Can you work these out from the drawing? Everything is in mm from the part's minimum corner. A direction names the side the tool comes from. Round coordinates to 2 decimals unless told otherwise and drop trailing zeros. Write each loop counter-clockwise with the first axis right and the second up, starting at its lowest first coordinate (ties: lowest second). Pieces come first, ordered by that corner, then holes. Notation, with made-up numbers: (-3, 47) -> (2, 47) arc R12 ccw to (2, 53) -> close; hole circle Ø11 at (30.25, 12.5). An arc over 180 degrees is marked (long way). Answer as CSV lines item,"result". Start each with the question number.
Q1. For the marked faces 1 and 2, which set-ups out of +Z, -Z, +X, -X, +Y, -Y let a thin tool reach every point of the face, with its end or its side?
Q2. Imagine slicing it at B-B on x = 10.5. Please give me the cut outline in (y, z).
Q3. Imagine slicing it at C-C on z = 5.25. Please give me the cut outline in (x, y).
Q4. Imagine slicing it at A-A on y = 2.25. Please give me the cut outline in (x, z).
Q5. If I drill on line 1 (Z direction, x = 5.5, y = 10); line 2 (X direction, y = 17.5, z = 2.5); line 3 (Z direction, x = 2.25, y = 3.75) (1 decimal), over which ranges is the centre line in solid material (lowest first)? Write a range as [from, to].
Q6. Will these pins go through, and if not, where does the flat tip stop? pin 1 Ø4.5 at (y, z) = (7, 6) entering from +X; pin 2 Ø1.5 at (x, y) = (8.5, 2.5) entering from -Z.
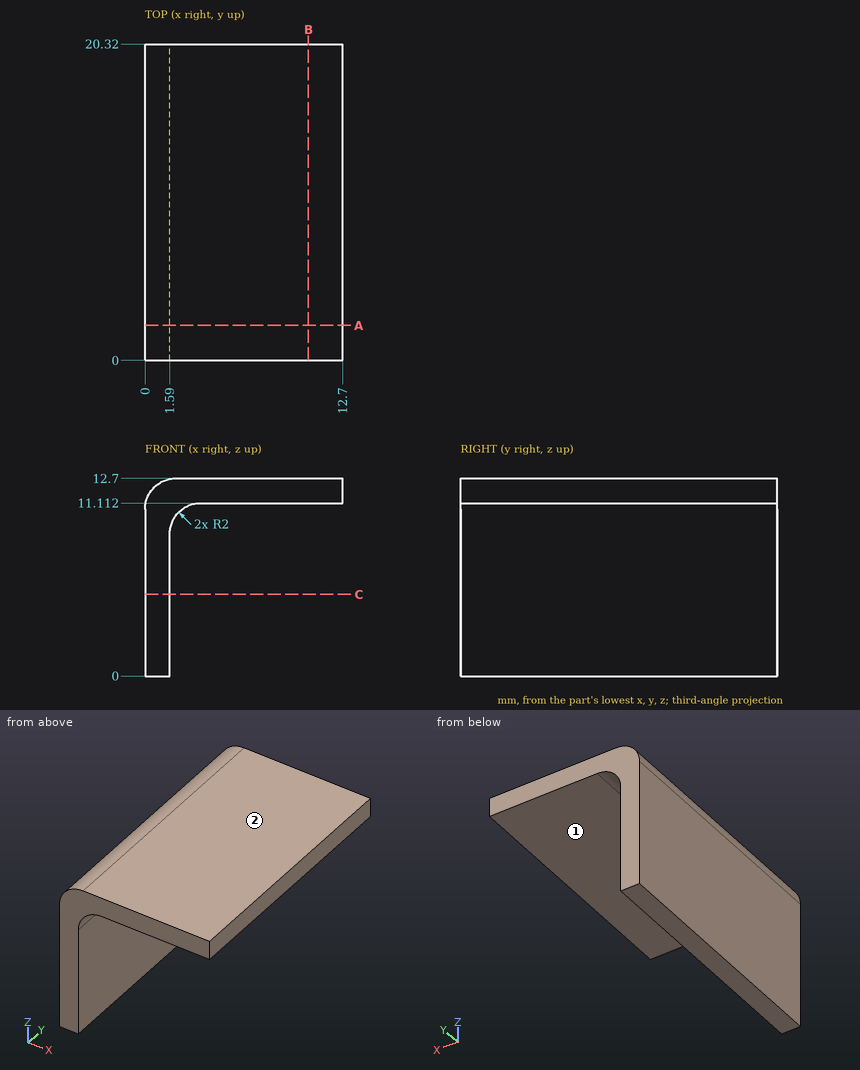
Checks:
1,face 1,"-Z, +X, +Y, -Y"
1,face 2,"+Z, +X, -X, +Y, -Y"
2,outline,"(0, 11.11) -> (20.32, 11.11) -> (20.32, 12.7) -> (0, 12.7) -> close"
3,outline,"(0, 0) -> (1.59, 0) -> (1.59, 20.32) -> (0, 20.32) -> close"
4,outline,"(0, 0) -> (1.59, 0) -> (1.59, 9.11) arc R2 cw to (3.59, 11.11) -> (12.7, 11.11) -> (12.7, 12.7) -> (2, 12.7) arc R2 ccw to (0, 10.7) -> close"
5,line 1,"[11.11, 12.7]"
5,line 2,"[0, 1.59]"
5,line 3,"[10.6, 12.7]"
6,pin 1,"x = 1.59"
6,pin 2,"z = 11.11"
